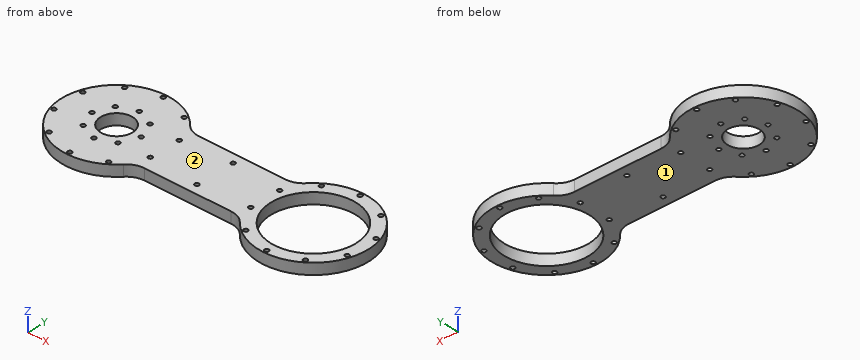
```python
from build123d import *

# Parameters (mm, degrees)
ESQUISSE1_W             = 320
ESQUISSE1_H             = 120
ESQUISSE1_R             = 42.5
ESQUISSE1_R_2           = 16
BOSS_EXTRU_1_DEPTH      = 11
ESQUISSE2_R             = 2.1
ENL_V_MAT_EXTRU_1_DEPTH = 268.05991837
ESQUISSE3_OUTSIDE_W     = 390.388
ESQUISSE3_OUTSIDE_H     = 190.388
ENL_V_MAT_EXTRU_2_DEPTH = 268.05991837
CONG_1_R                = 20
ESQUISSE4_R             = 2.1
ENL_V_MAT_EXTRU_3_DEPTH = 262.095767871
ESQUISSE5_R             = 2.1
ENL_V_MAT_EXTRU_4_DEPTH = 84


with BuildPart() as part:
    # Esquisse1 → Boss.-Extru.1 (new body)
    with BuildSketch(Plane.XY):
        with Locations((-100, 0)):
            Rectangle(ESQUISSE1_W, ESQUISSE1_H)
        Circle(ESQUISSE1_R, mode=Mode.SUBTRACT)
        with Locations((-200, 0)):
            Circle(ESQUISSE1_R_2, mode=Mode.SUBTRACT)
    extrude(amount=BOSS_EXTRU_1_DEPTH)

    # Esquisse2 → Enlèv. mat.-Extru.1 (cut, through all)
    with BuildSketch(Plane.XY.offset(11)):
        with Locations((-200, 25)):
            Circle(ESQUISSE2_R)
        with Locations((-182.32233047, 17.67766953)):
            Circle(ESQUISSE2_R)
        with Locations((-175, 0)):
            Circle(ESQUISSE2_R)
        with Locations((-182.32233047, -17.67766953)):
            Circle(ESQUISSE2_R)
        with Locations((-200, -25)):
            Circle(ESQUISSE2_R)
        with Locations((-217.67766953, -17.67766953)):
            Circle(ESQUISSE2_R)
        with Locations((-225, 0)):
            Circle(ESQUISSE2_R)
        with Locations((-217.67766953, 17.67766953)):
            Circle(ESQUISSE2_R)
    extrude(amount=-ENL_V_MAT_EXTRU_1_DEPTH, mode=Mode.SUBTRACT)

    # Esquisse3 outside → Enlèv. mat.-Extru.2 (cut, through all)
    with BuildSketch(Plane.XY.offset(11)):
        with Locations((-100, 0)):
            Rectangle(ESQUISSE3_OUTSIDE_W, ESQUISSE3_OUTSIDE_H)
        with BuildLine():
            Line((-153.902277714, 30), (-46.097722286, 30))
            ThreePointArc((-46.097722286, 30), (55, 0), (-46.097722286, -30))
            Line((-46.097722286, -30), (-153.902277714, -30))
            ThreePointArc((-153.902277714, -30), (-255, 0), (-153.902277714, 30))
        make_face(mode=Mode.SUBTRACT)
    extrude(amount=-ENL_V_MAT_EXTRU_2_DEPTH, mode=Mode.SUBTRACT)

    # Congé1
    cong_1_edges = [part.edges().sort_by_distance(p)[0] for p in [
        (-153.902277714, 30, 5.5),
        (-46.097722286, 30, 5.5),
        (-46.097722286, -30, 5.5),
        (-153.902277714, -30, 5.5),
    ]]
    fillet(cong_1_edges, radius=CONG_1_R)

    # Esquisse4 → Enlèv. mat.-Extru.3 (cut, through all)
    with BuildSketch(Plane.XY.offset(11)):
        with Locations((-200, 51.5)):
            Circle(ESQUISSE4_R)
        with Locations((-169.729059507, 41.66437521)):
            Circle(ESQUISSE4_R)
        with Locations((-151.020589411, 15.91437521)):
            Circle(ESQUISSE4_R)
        with Locations((-151.020589411, -15.91437521)):
            Circle(ESQUISSE4_R)
        with Locations((-169.729059507, -41.66437521)):
            Circle(ESQUISSE4_R)
        with Locations((-200, -51.5)):
            Circle(ESQUISSE4_R)
        with Locations((-230.270940493, -41.66437521)):
            Circle(ESQUISSE4_R)
        with Locations((-248.979410589, -15.91437521)):
            Circle(ESQUISSE4_R)
        with Locations((-248.979410589, 15.91437521)):
            Circle(ESQUISSE4_R)
        with Locations((-230.270940493, 41.66437521)):
            Circle(ESQUISSE4_R)
        with Locations(Location((30.270940493, 41.66437521, 0), (0, 0, 180))):
            Circle(ESQUISSE4_R)
        with Locations(Location((48.979410589, 15.91437521, 0), (0, 0, 180))):
            Circle(ESQUISSE4_R)
        with Locations(Location((48.979410589, -15.91437521, 0), (0, 0, 180))):
            Circle(ESQUISSE4_R)
        with Locations(Location((30.270940493, -41.66437521, 0), (0, 0, 180))):
            Circle(ESQUISSE4_R)
        with Locations(Location((0, -51.5, 0), (0, 0, 180))):
            Circle(ESQUISSE4_R)
        with Locations(Location((-30.270940493, -41.66437521, 0), (0, 0, 180))):
            Circle(ESQUISSE4_R)
        with Locations(Location((-48.979410589, -15.91437521, 0), (0, 0, 180))):
            Circle(ESQUISSE4_R)
        with Locations(Location((-48.979410589, 15.91437521, 0), (0, 0, 180))):
            Circle(ESQUISSE4_R)
        with Locations(Location((-30.270940493, 41.66437521, 0), (0, 0, 180))):
            Circle(ESQUISSE4_R)
        with Locations(Location((0, 51.5, 0), (0, 0, 180))):
            Circle(ESQUISSE4_R)
    extrude(amount=-ENL_V_MAT_EXTRU_3_DEPTH, mode=Mode.SUBTRACT)

    # Esquisse5 → Enlèv. mat.-Extru.4 (cut)
    with BuildSketch(Plane.XY.offset(11)):
        with Locations((-100, 20)):
            Circle(ESQUISSE5_R)
        with Locations((-100, -20)):
            Circle(ESQUISSE5_R)
    extrude(amount=-ENL_V_MAT_EXTRU_4_DEPTH, mode=Mode.SUBTRACT)


solid = part.part
```
Check sheet for the modelled part. Datum: model origin and axes. Units: mm. Face numbers are marked on the shaded views. Round coordinates to 2 decimals unless told otherwise and drop trailing zeros. Order: outer loops, then holes, each group sorted by start corner. A loop starts at its lowest first (then second) coordinate and runs counter-clockwise, first axis right, second up.
1) Section check C-C (x = -75). Record the boundary of the cut face in (y, z), and give its area (3 significant figures).
2) Go/stop test with flat-tipped pins: pin 1 Ø4 at (x, y) = (-90.5, 14.5) entering from -Z; pin 2 Ø4 at (x, y) = (48.98, 15.91) entering from +Z; pin 3 Ø1.5 at (y, z) = (-34.5, 6.5) entering from +X; pin 4 Ø1.5 at (y, z) = (0.5, 6) entering from +X. Record where each tip stops, or that it passes through.
3) Section check D-D (z = 5). Give the number of separate pieces and of enclosed holes in the cut face, and give its area (3 significant figures).
4) Section check A-A (y = 11). Record the boundary of the cut face in (x, z), and give its area (3 significant figures).
5) Scan lines: line 1 (Y direction, x = 0, z = 6.5); line 2 (X direction, y = 50, z = 6.25); line 3 (X direction, y = -36, z = 6.5). Record each from-to range of solid material in increasing order.
6) Mould release check, pull along Z, two halves, no side actions. Record for the marked faces 1 and 2: +Z half, -Z half, draft (parallel to the pull), parting line (faces both ways), or undercut.
7) Section check B-B (x = -6). Record the boundary of the cut face in (y, z).
Result:
1. outline: (-30, 0) - (30, 0) - (30, 11) - (-30, 11) - close
1. area: 660 mm2
2. pin 1: stops at z = 0
2. pin 2: passes through
2. pin 3: stops at x = 43.43
2. pin 4: stops at x = 55
3. separate pieces: 1
3. enclosed holes: 32
3. area: 17,900 mm2
4. outline: (-253.89, 0) - (-211.62, 0) - (-211.62, 11) - (-253.89, 11) - close; (-188.38, 0) - (-41.05, 0) - (-41.05, 11) - (-188.38, 11) - close; (41.05, 0) - (53.89, 0) - (53.89, 11) - (41.05, 11) - close
4. area: 2,230 mm2
5. line 1: y = -55 to -53.6, -49.4 to -42.5, 42.5 to 49.4, 53.6 to 55
5. line 2: x = -222.91 to -201.47, -198.53 to -177.09, -22.91 to -1.47, 1.47 to 22.91
5. line 3: x = -241.58 to -158.38, -41.62 to -22.59, 22.59 to 41.58
6. face 1: -Z half
6. face 2: +Z half
7. outline: (-54.67, 0) - (-42.07, 0) - (-42.07, 11) - (-54.67, 11) - close; (42.07, 0) - (54.67, 0) - (54.67, 11) - (42.07, 11) - close
